```python
from build123d import *

# Parameters (mm, degrees)
F0_W        = 200
F0_H        = 80
F1_DEPTH    = 30
F2_W        = 60
F2_H        = 25
F3_DEPTH    = 10
F4_W        = 60
F4_H        = 25
F5_DEPTH    = 10
F6_T1_DEPTH = 41.75
F6_T3_DEPTH = 41.75


# Not quite as in the source:
# - a fillet or chamfer that OpenCascade refuses, or shapes differently, is made with other operations: its cross-section is extruded or revolved along the edge and cut away or added


with BuildPart() as f1:
    # F0 (on Top) → F1 (new body)
    with BuildSketch(Plane.XY):
        Rectangle(F0_W, F0_H)
    extrude(amount=F1_DEPTH)

    # F2 (on face) → F3 (join)
    with BuildSketch(Plane(origin=(-100, 0, 0), x_dir=(0, -1, 0), z_dir=(-1, 0, 0))):
        with Locations((0, 15)):
            Rectangle(F2_W, F2_H)
    extrude(amount=F3_DEPTH)

    # F4 (on face) → F5 (join)
    with BuildSketch(Plane.YZ.offset(100)):
        with Locations((0, 15)):
            Rectangle(F4_W, F4_H)
    extrude(amount=F5_DEPTH)

    # F6: fillet of radius 12.7 on 8 edges, made by hand

    # F6_s2 → F6_t1 (cut)
    with BuildSketch(Plane.YZ.offset(100)):
        with BuildLine():
            ThreePointArc((-30, 14.8), (-26.2802561211, 23.7802561211), (-17.3, 27.5))
            Line((-17.3, 27.5), (-30, 27.5))
            Line((-30, 27.5), (-30, 14.8))
        make_face()
        with BuildLine():
            ThreePointArc((-30, 15.2), (-26.2802561211, 6.2197438789), (-17.3, 2.5))
            Line((-17.3, 2.5), (-30, 2.5))
            Line((-30, 2.5), (-30, 15.2))
        make_face()
        with BuildLine():
            ThreePointArc((17.3, 27.5), (26.2802561211, 23.7802561211), (30, 14.8))
            Line((30, 14.8), (30, 27.5))
            Line((30, 27.5), (17.3, 27.5))
        make_face()
        with BuildLine():
            ThreePointArc((30, 15.2), (26.2802561211, 6.2197438789), (17.3, 2.5))
            Line((17.3, 2.5), (30, 2.5))
            Line((30, 2.5), (30, 15.2))
        make_face()
    extrude(amount=F6_T1_DEPTH, mode=Mode.SUBTRACT)

    # F6_s4 → F6_t3 (cut)
    with BuildSketch(Plane.YZ.offset(-141.75)):
        with BuildLine():
            ThreePointArc((30, 14.8), (26.2802561211, 23.7802561211), (17.3, 27.5))
            Line((17.3, 27.5), (30, 27.5))
            Line((30, 27.5), (30, 14.8))
        make_face()
        with BuildLine():
            ThreePointArc((-17.3, 27.5), (-26.2802561211, 23.7802561211), (-30, 14.8))
            Line((-30, 14.8), (-30, 27.5))
            Line((-30, 27.5), (-17.3, 27.5))
        make_face()
        with BuildLine():
            ThreePointArc((-17.3, 2.5), (-26.2802561211, 6.2197438789), (-30, 15.2))
            Line((-30, 15.2), (-30, 2.5))
            Line((-30, 2.5), (-17.3, 2.5))
        make_face()
        with BuildLine():
            ThreePointArc((17.3, 2.5), (26.2802561211, 6.2197438789), (30, 15.2))
            Line((30, 15.2), (30, 2.5))
            Line((30, 2.5), (17.3, 2.5))
        make_face()
    extrude(amount=F6_T3_DEPTH, mode=Mode.SUBTRACT)


solid = f1.part
```
Input: part model. Units: mm. Frame: model coordinates. A direction names the side the tool comes from. Coordinates: 2 decimals unless noted, no trailing zeros. Write each loop counter-clockwise with the first axis right and the second up, starting at its lowest first coordinate (ties: lowest second). Pieces come first, ordered by that corner, then holes. Notation, with made-up numbers: (74, -15) -> (85, -15) arc R21 ccw to (85, -8) -> close; hole circle Ø11 at (73, 29.25). An arc over 180 degrees is marked (long way). Answer as a JSON object with one key per item and string values.
1. Access query for faces 1 (the face through (-105.07, -26.11, 23.95)), 2 (the face through (105, 0, 2.5)), 3 (the face through (-105, 0, 27.5)). Directions: +Z, -Z, +X, -X, +Y, -Y. A direction counts if a zero-diameter tool reaches every point of the face in a straight line with its end or side. Return the directions, or none.
Result set:
{"face 1": "+Z, -X, -Y", "face 2": "-Z, +X, +Y, -Y", "face 3": "+Z, -X, +Y, -Y"}
2. Section A-A on y = 24. Return the cut outline in (x, z), then the cut area to 3 significant figures.
Result set:
{"outline": "(-110, 4.41) -> (-100, 4.41) -> (-100, 0) -> (100, 0) -> (100, 4.41) -> (110, 4.41) -> (110, 25.59) -> (100, 25.59) -> (100, 30) -> (-100, 30) -> (-100, 25.59) -> (-110, 25.59) -> close", "area": "6,420 mm2"}
3. Section B-B on z = 9. Return the cut outline in (x, y), then the cut area to 3 significant figures.
Result set:
{"outline": "(-110, -28.38) -> (-100, -28.38) -> (-100, -40) -> (100, -40) -> (100, -28.38) -> (110, -28.38) -> (110, 28.38) -> (100, 28.38) -> (100, 40) -> (-100, 40) -> (-100, 28.38) -> (-110, 28.38) -> close", "area": "17,100 mm2"}
4. First-contact query: P1, Ø8, axis at x = -106, y = 1, coming from the -Z side; P2, Ø8, axis at x = 106.5, y = 7, coming from the +Z side. Flat tips, straight axial feed; report the tip coordinate or a pass-through.
Result set:
{"P1": "stops at z = 2.5", "P2": "stops at z = 27.5"}
5. Material intervals for line 1 (X direction, y = 33.5, z = 18.75), sorted ascending. Write a range as from..to.
Result set:
{"line 1": "x = -100..100"}
